The model under review builds one solid part; all positions refer to its coordinate system, in mm. Coordinates: 2 decimals unless noted, no trailing zeros. Loops run counter-clockwise (first coordinate to the right, second up) from the corner with the lowest first, then second, coordinate; pieces in that order, holes last. Notation, with made-up numbers: M -31,23.5 L -27,23.5 A28 cw -27,59.5 Z; hole C 1.5,85 d6. An arc over 180 degrees is marked long. Write item = value, one per line. Start each with the question number.
Q1. Wall thickness on probe 1 along Y at (x, z) = (-55, 3.05); probe 2 along Y at (x, z) = (-16, 3.5); probe 3 along X at (y, z) = (-16.5, 2.25): over which ranges is each line inside the solid? List them lowest first.
Q2. We need section A-A on x = 71. Give the boundary of the cut face in (y, z).
Q3. We need section B-B on x = -16. Give the boundary of the cut face in (y, z).
Q4. We need section C-C on z = 0.9. Count the separate pieces of the cut face and the enclosed holes in it, and give its area (3 significant figures).
Q5. Mouldability with a two-part tool opening along Y and no side actions: class faces 1 (the face through (-85, 0, 2)), 2 (the face through (-1, 21, 2)), 3 (the face through (36.752, 0.099, 2.535)) as released by +Y, released by -Y, zero draft, split by the parting line, or undercut.
from build123d import *

# Parameters (mm, degrees)
SKETCH1_W               = 170
SKETCH1_H               = 42
BOSS_EXTRUDE1_DEPTH     = 5
CUT_EXTRUDE1_DEPTH      = 88.698346621
CUT_EXTRUDE1_DEPTH_BACK = 88.698346621
SKETCH2_R               = 6.1
CUT_EXTRUDE2_DEPTH      = 88.698346621
CUT_EXTRUDE2_DEPTH_BACK = 88.698346621
SKETCH3_R               = 3
SKETCH4_R               = 2.25
CUT_EXTRUDE3_DEPTH      = 88.698346621


with BuildPart() as part:
    # Sketch1 → Boss-Extrude1 (new body)
    with BuildSketch(Plane.XY):
        Rectangle(SKETCH1_W, SKETCH1_H)
    extrude(amount=BOSS_EXTRUDE1_DEPTH)

    # Sketch2 → Cut-Extrude1 (cut, two sides: drawn at the far end of the back side and taken through both)
    with BuildSketch(Plane.XY.offset(5).offset(-CUT_EXTRUDE1_DEPTH_BACK)):
        with Locations((-55, 0)):
            Circle(SKETCH2_R)
        with Locations((55, 0)):
            Circle(SKETCH2_R)
    extrude(amount=CUT_EXTRUDE1_DEPTH + CUT_EXTRUDE1_DEPTH_BACK, mode=Mode.SUBTRACT)

    # Sketch3 → Cut-Extrude2 (cut, two sides: drawn at the far end of the back side and taken through both)
    with BuildSketch(Plane.XY.offset(5).offset(-CUT_EXTRUDE2_DEPTH_BACK)):
        with Locations((-16, -12.5)):
            Circle(SKETCH3_R)
        with Locations((-16, 12.5)):
            Circle(SKETCH3_R)
        with Locations((16, 12.5)):
            Circle(SKETCH3_R)
        with Locations((16, -12.5)):
            Circle(SKETCH3_R)
    extrude(amount=CUT_EXTRUDE2_DEPTH + CUT_EXTRUDE2_DEPTH_BACK, mode=Mode.SUBTRACT)

    # Sketch4 → Cut-Extrude3 (cut, through all)
    with BuildSketch(Plane.XY.offset(5)):
        with Locations((-71, 0)):
            Circle(SKETCH4_R)
        with Locations((-55, 16)):
            Circle(SKETCH4_R)
        with Locations((-39, 0)):
            Circle(SKETCH4_R)
        with Locations((-55, -16)):
            Circle(SKETCH4_R)
        with Locations((39, 0)):
            Circle(SKETCH4_R)
        with Locations((55, 16)):
            Circle(SKETCH4_R)
        with Locations((71, 0)):
            Circle(SKETCH4_R)
        with Locations((55, -16)):
            Circle(SKETCH4_R)
    extrude(amount=-CUT_EXTRUDE3_DEPTH, mode=Mode.SUBTRACT)


solid = part.part
Returned:
q1.probe_1 = -21 to -18.25, -13.75 to -6.1, 6.1 to 13.75, 18.25 to 21
q1.probe_2 = -21 to -15.5, -9.5 to 9.5, 15.5 to 21
q1.probe_3 = -85 to -57.19, -52.81 to 52.81, 57.19 to 85
q2.outline = M -21,0 L -2.25,0 L -2.25,5 L -21,5 Z; M 2.25,0 L 21,0 L 21,5 L 2.25,5 Z
q3.outline = M -21,0 L -15.5,0 L -15.5,5 L -21,5 Z; M -9.5,0 L 9.5,0 L 9.5,5 L -9.5,5 Z; M 15.5,0 L 21,0 L 21,5 L 15.5,5 Z
q4.separate_pieces = 1
q4.enclosed_holes = 14
q4.area = 6,670 mm^2
q5.face_1 = zero draft
q5.face_2 = released by +Y
q5.face_3 = undercut
